Can you work these out from the model? Positions are in its coordinate system, mm. Give positions to 0.01 mm unless a question says otherwise; leave off trailing zeros. Order: outer loops, then holes, each group sorted by start corner. A loop starts at its lowest first (then second) coordinate and runs counter-clockwise, first axis right, second up. Notation, with made-up numbers: (-29, -7) - (-13, -7) arc R5 cw to (-13, 1) - close; hole circle Ø7 at (-13, 30). An arc over 180 degrees is marked (long way). Return JSON: item names as keys, results as strings.
```python
from build123d import *

# Parameters (mm, degrees)
SKETCH_1_W          = 60
SKETCH_1_H          = 30
EXTRUDE_1_DEPTH     = 3
SKETCH_2_R          = 1.75
CUT_EXTRUDE_2_DEPTH = 54.935146241


with BuildPart() as part:
    # 草圖1 → 伸長1 (new body)
    with BuildSketch(Plane.XY):
        with Locations((-20, 5)):
            Rectangle(SKETCH_1_W, SKETCH_1_H)
    extrude(amount=EXTRUDE_1_DEPTH)

    # 草圖2 → 伸長2 (cut, through all)
    with BuildSketch(Plane.XY.offset(3)):
        with Locations((-40, 0)):
            Circle(SKETCH_2_R)
        Circle(SKETCH_2_R)
    extrude(amount=-CUT_EXTRUDE_2_DEPTH, mode=Mode.SUBTRACT)


solid = part.part
```
1. Suppose I cut it at C-C (x = 1). List the corners of the cut face in (y, z) for me, plus the area to 3 significant figures.
Checks:
{"outline": "(-10, 0) - (-1.44, 0) - (-1.44, 3) - (-10, 3) - close; (1.44, 0) - (20, 0) - (20, 3) - (1.44, 3) - close", "area": "81.4 mm^2"}
2. Suppose I cut it at A-A (y = 0). List the corners of the cut face in (x, z) for me.
Checks:
{"outline": "(-50, 0) - (-41.75, 0) - (-41.75, 3) - (-50, 3) - close; (-38.25, 0) - (-1.75, 0) - (-1.75, 3) - (-38.25, 3) - close; (1.75, 0) - (10, 0) - (10, 3) - (1.75, 3) - close"}
3. If I drill on L1, parallel to X at y = 0.5, z = 0.3; L2, parallel to Y at x = 0, z = 1.15; L3, parallel to X at y = 1.25, z = 2.1, over which ranges is the centre line in solid material (lowest first)? Write a range as [from, to].
Checks:
{"L1": "[-50, -41.68], [-38.32, -1.68], [1.68, 10]", "L2": "[-10, -1.75], [1.75, 20]", "L3": "[-50, -41.22], [-38.78, -1.22], [1.22, 10]"}
4. For pin 1 Ø3 at (x, y) = (0, 0) entering from +Z, with a flat end and sliding along its axis, tell me the tip position at first contact or that it passes through.
Checks:
{"pin 1": "through"}
5. Suppose I cut it at B-B (x = -40). List the corners of the cut face in (y, z) for me.
Checks:
{"outline": "(-10, 0) - (-1.75, 0) - (-1.75, 3) - (-10, 3) - close; (1.75, 0) - (20, 0) - (20, 3) - (1.75, 3) - close"}
6. Thinking about a two-plate mould opening in X: for faces 1 (the face through (10, 5, 1)), 2 (the face through (-38.383, -0.67, 1.521)), 3 (the face through (-50, 5, 1)), 4 (the face through (-20, -10, 1)), which applies, +X half, -X half, draft (parallel to the pull), parting line (faces both ways), or undercut?
Checks:
{"face 1": "+X half", "face 2": "undercut", "face 3": "-X half", "face 4": "draft"}
